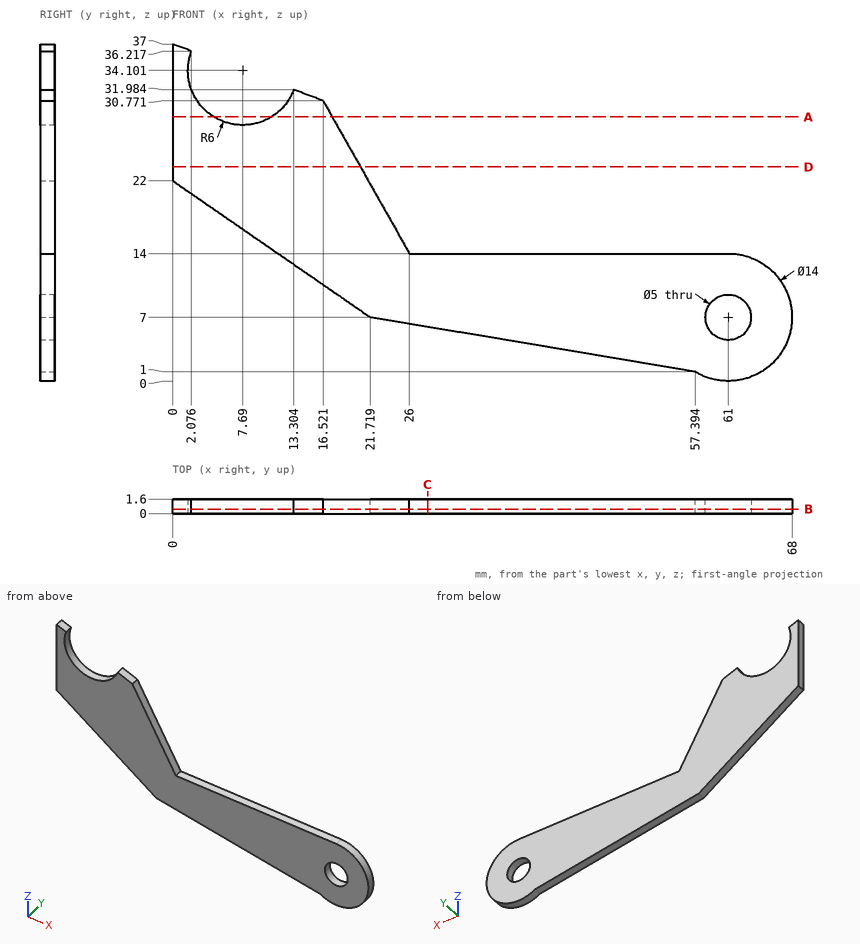
Geometry: see drawing. Coordinates: mm, zero at the bounding-box minimum. Coordinates: 2 decimals unless noted, no trailing zeros. Order: outer loops, then holes, each group sorted by start corner. A loop starts at its lowest first (then second) coordinate and runs counter-clockwise, first axis right, second up. Notation, with made-up numbers: (-30.5, -12.5) - (24.5, -12.5) arc R21 ccw to (24.5, 17.5) - close; hole circle Ø1 at (22.25, 32.25). An arc over 180 degrees is marked (long way). Use one line per item in the form item = value.
1) Section A-A (z = 29). Return loops of the section in (x, y).
Solutions:
outline = (0, 0) - (4.53, 0) - (4.53, 1.6) - (0, 1.6) - close; (10.85, 0) - (17.52, 0) - (17.52, 1.6) - (10.85, 1.6) - close
2) Section C-C (x = 28). Return loops of the section in (y, z), then the cut area to 3 significant figures.
Solutions:
outline = (0, 5.94) - (1.6, 5.94) - (1.6, 14) - (0, 14) - close
area = 12.9 mm^2
3) Section D-D (z = 23.5). Return loops of the section in (x, y).
Solutions:
outline = (0, 0) - (20.63, 0) - (20.63, 1.6) - (0, 1.6) - close
4) Ray query, L1, parallel to Z at x = 61, y = 1.15; L2, parallel to Z at x = 36.5, y = 0.6 (1 decimal); L3, parallel to Z at x = 62.5, y = 1.35 (1 decimal). Return the intervals inside material, ascending.
Solutions:
L1 = 0 to 4.5, 9.5 to 14
L2 = 4.5 to 14
L3 = 0.2 to 5, 9 to 13.8
5) Section B-B (y = 0.5). Return loops of the section in (x, z) (1 decimal), then the cut area to 3 significant figures.
Solutions:
outline = (0, 22) - (21.7, 7) - (57.4, 1) arc R7 ccw (long way) to (61, 14) - (26, 14) - (16.5, 30.8) - (13.3, 32) arc R6 cw to (2.1, 36.2) - (0, 37) - close; hole circle Ø5 at (61, 7)
area = 804 mm^2
